Verification items for the finished model (mm, model axes). A direction names the side the tool comes from. Give positions to 0.01 mm unless a question says otherwise; leave off trailing zeros. Write each loop counter-clockwise with the first axis right and the second up, starting at its lowest first coordinate (ties: lowest second). Pieces come first, ordered by that corner, then holes.
from build123d import *

# Parameters (mm, degrees)
SKETCH1_R           = 9.525
BOSS_EXTRUDE1_DEPTH = 0.409575


with BuildPart() as part:
    # Sketch1 → Boss-Extrude1 (new, symmetric)
    with BuildSketch(Plane.XY):
        with Locations(Location((0, 0, 0), (0, 0, 180))):
            Circle(SKETCH1_R)
        Polygon((0, 7.332348419), (-6.35, 3.666174209), (-6.35, -3.666174209), (0, -7.332348419), (6.35, -3.666174209), (6.35, 3.666174209), align=None, mode=Mode.SUBTRACT)
    extrude(amount=BOSS_EXTRUDE1_DEPTH, both=True)


solid = part.part
Item 1: Sectioned sample at C-C on z = 0. Record the cut outline in (x, y) (3 decimals).
Answer key:
outline: circle Ø19.05 at (0, 0); hole (-6.35, -3.666) - (0, -7.332) - (6.35, -3.666) - (6.35, 3.666) - (0, 7.332) - (-6.35, 3.666) - close
Item 2: Sectioned sample at B-B on x = 3.25. Record the cut outline in (y, z).
Answer key:
outline: (-8.95, -0.41) - (-5.46, -0.41) - (-5.46, 0.41) - (-8.95, 0.41) - close; (5.46, -0.41) - (8.95, -0.41) - (8.95, 0.41) - (5.46, 0.41) - close
Item 3: Scan lines: line 1 along X through (y, z) = (1.75, 0.25); line 2 along X through (y, z) = (-5.5, 0); line 3 along Y through (x, z) = (2.25, 0.3). Record each from-to range of solid material in increasing order.
Answer key:
line 1: x = -9.36 to -6.35, 6.35 to 9.36
line 2: x = -7.78 to -3.17, 3.17 to 7.78
line 3: y = -9.26 to -6.03, 6.03 to 9.26
Item 4: Release check for a two-part mould opening along X. For faces 3 (the face through (2.06, 9.3, 0.01)), 4 (the face through (-6.35, 0, 0)), 5 (the face through (2.3, 6.2, -0.41)) record: released by +X, released by -X, zero draft, split by the parting line, or undercut.
Answer key:
face 3: split by the parting line
face 4: undercut
face 5: zero draft
Item 5: Set-up check for faces 1 (the face through (2.3, 6.2, 0.41)), 2 (the face through (-3.131, 5.525, 0.006)): record each of +Z, -Z, +X, -X, +Y, -Y from which the full face is reachable in a straight line by a thin tool's end or side.
Answer key:
face 1: +Z, +X, -X, +Y, -Y
face 2: +Z, -Z
Item 6: Sectioned sample at D-D on x = 6.75. Record the cut outline in (y, z), then the cut area to 3 significant figures.
Answer key:
outline: (-6.72, -0.41) - (6.72, -0.41) - (6.72, 0.41) - (-6.72, 0.41) - close
area: 11.0 mm2
Item 7: Sectioned sample at A-A on y = -4.75. Record the cut outline in (x, z).
Answer key:
outline: (-8.26, -0.41) - (-4.47, -0.41) - (-4.47, 0.41) - (-8.26, 0.41) - close; (4.47, -0.41) - (8.26, -0.41) - (8.26, 0.41) - (4.47, 0.41) - close
